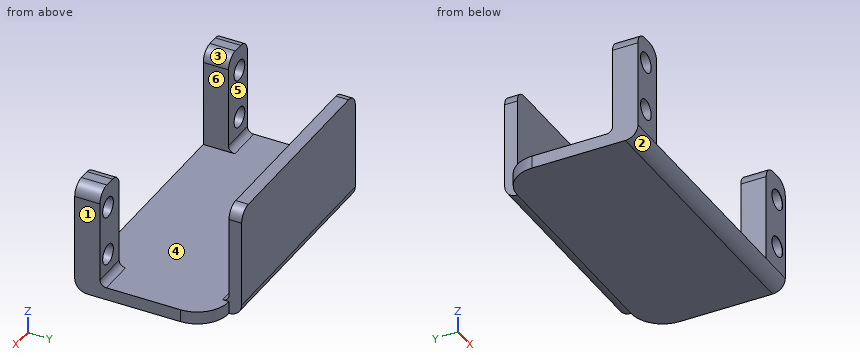
from build123d import *

# Parameters (mm, degrees)
SKETCH2_W                      = 42.8
SKETCH2_H                      = 2.54
BOSS_EXTRUDE1_DEPTH            = 2.54
SKETCH7_W                      = 7.192
SKETCH7_H                      = 5.08
SKETCH7_W_2                    = 42.8
SKETCH7_H_2                    = 2.54
BOSS_EXTRUDE3_DEPTH            = 20
FILLET3_R                      = 2.54
FILLET4_R                      = 1.27
CUT_EXTRUDE2_REACH             = 49.098
SKETCH8_R                      = 2.01
CUT_EXTRUDE2_DIRECTION_2_REACH = 49.098


# Some blends are built 0.0001 mm under size
with BuildPart() as part:
    # Sketch2 → Boss-Extrude1 (new body)
    with BuildSketch(Plane.XY):
        with Locations((-2.467346939, 15.826258503)):
            Rectangle(SKETCH2_W, SKETCH2_H)
        with BuildLine():
            Line((18.932653061, 14.556258503), (-23.867346939, 14.556258503))
            ThreePointArc((-23.867346939, 14.556258503), (-28.357474999, 12.696386564), (-30.217346939, 8.206258503))
            Line((-30.217346939, 8.206258503), (-30.217346939, -13.013741497))
            Line((-30.217346939, -13.013741497), (25.282653061, -13.013741497))
            Line((25.282653061, -13.013741497), (25.282653061, 8.206258503))
            ThreePointArc((25.282653061, 8.206258503), (23.422781122, 12.696386564), (18.932653061, 14.556258503))
        make_face()
    extrude(amount=-BOSS_EXTRUDE1_DEPTH)

    # Sketch7 → Boss-Extrude3 (add)
    with BuildSketch(Plane.XY):
        Polygon((-30.217346939, -7.933741497), (-30.217346939, -13.013741497), (-23.125346939, -13.003741497), (-23.125346939, -7.933741497), align=None)
        with Locations((21.686653061, -10.473741497)):
            Rectangle(SKETCH7_W, SKETCH7_H)
        with Locations((-2.467346939, 15.826258503)):
            Rectangle(SKETCH7_W_2, SKETCH7_H_2)
    extrude(amount=BOSS_EXTRUDE3_DEPTH)

    # Fillet3
    fillet3_edges = [part.edges().sort_by_distance(p)[0] for p in [
        (-2.467346939, 17.096258503, -2.54),
        (18.932653061, 15.826258503, 20),
        (-23.867346939, 15.826258503, 20),
        (-2.467346939, -13.013741497, -2.54),
        (18.090653061, -10.473741497, 20),
        (25.282653061, -10.473741497, 20),
        (-23.125346939, -10.468741497, 20),
        (-30.217346939, -10.473741497, 20),
    ]]
    fillet(fillet3_edges, radius=FILLET3_R - 0.0001)  # a hair under: the kernel refuses the full size

    # Fillet4
    # the kernel refuses this fillet: 1.27 mm, written as the material it adds along each edge
    with BuildSketch(Plane(origin=(-23.125346939, -7.933741497, 0), x_dir=(0, 1, 0), z_dir=(-1, 0, 0))) as fillet4_piece_1:
        with BuildLine():
            CenterArc((FILLET4_R, -FILLET4_R), FILLET4_R, 90, 90)
            Line((0, -FILLET4_R), (0, 0))
            Line((0, 0), (FILLET4_R, 0))
        make_face()
    extrude(amount=7.092)
    with BuildSketch(Plane(origin=(25.282653061, -7.933741497, 0), x_dir=(0, 1, 0), z_dir=(-1, 0, 0))) as fillet4_piece_2:
        with BuildLine():
            CenterArc((FILLET4_R, -FILLET4_R), FILLET4_R, 90, 90)
            Line((0, -FILLET4_R), (0, 0))
            Line((0, 0), (FILLET4_R, 0))
        make_face()
    extrude(amount=7.192)
    with BuildSketch(Plane(origin=(-23.867346939, 14.556258503, 0), x_dir=(0, 0, 1), z_dir=(1, 0, 0))) as fillet4_piece_3:
        with BuildLine():
            CenterArc((FILLET4_R, FILLET4_R), FILLET4_R, 180, 90)
            Line((0, FILLET4_R), (0, 0))
            Line((0, 0), (FILLET4_R, 0))
        make_face()
    extrude(amount=42.8)

    # Cut-Extrude2: up to this face of the body (flat: up to its plane)
    cut_extrude2_end = Plane(part.part.faces().sort_by_distance((-26.671346939, -7.933741497, 10.447713694))[0])
    # Sketch8 → Cut-Extrude2 (cut, up to the picked face)
    with BuildSketch(Plane(origin=(0.018289774, -12.971108055, 0), x_dir=(0.9999990058958133, 0.0014100380793790163, 0), z_dir=(0.0014100380793790163, -0.9999990058958133, 0)), mode=Mode.PRIVATE) as cut_extrude2_sk1:
        with Locations((-27.239885767, 5)):
            Circle(SKETCH8_R)
    cut_extrude2_tool1 = split(extrude(cut_extrude2_sk1.sketch, amount=-CUT_EXTRUDE2_REACH, mode=Mode.PRIVATE), bisect_by=cut_extrude2_end, keep=Keep.BOTH, mode=Mode.PRIVATE)
    # Sketch8 → Cut-Extrude2 (cut, up to the picked face)
    with BuildSketch(Plane(origin=(0.018289774, -12.971108055, 0), x_dir=(0.9999990058958133, 0.0014100380793790163, 0), z_dir=(0.0014100380793790163, -0.9999990058958133, 0)), mode=Mode.PRIVATE) as cut_extrude2_sk2:
        with Locations((22.260065025, 5)):
            Circle(SKETCH8_R)
    cut_extrude2_tool2 = split(extrude(cut_extrude2_sk2.sketch, amount=-CUT_EXTRUDE2_REACH, mode=Mode.PRIVATE), bisect_by=cut_extrude2_end, keep=Keep.BOTH, mode=Mode.PRIVATE)
    # Sketch8 → Cut-Extrude2 (cut, up to the picked face)
    with BuildSketch(Plane(origin=(0.018289774, -12.971108055, 0), x_dir=(0.9999990058958133, 0.0014100380793790163, 0), z_dir=(0.0014100380793790163, -0.9999990058958133, 0)), mode=Mode.PRIVATE) as cut_extrude2_sk3:
        with Locations((22.260065025, 15)):
            Circle(SKETCH8_R)
    cut_extrude2_tool3 = split(extrude(cut_extrude2_sk3.sketch, amount=-CUT_EXTRUDE2_REACH, mode=Mode.PRIVATE), bisect_by=cut_extrude2_end, keep=Keep.BOTH, mode=Mode.PRIVATE)
    # Sketch8 → Cut-Extrude2 (cut, up to the picked face)
    with BuildSketch(Plane(origin=(0.018289774, -12.971108055, 0), x_dir=(0.9999990058958133, 0.0014100380793790163, 0), z_dir=(0.0014100380793790163, -0.9999990058958133, 0)), mode=Mode.PRIVATE) as cut_extrude2_sk4:
        with Locations((-27.239885767, 15)):
            Circle(SKETCH8_R)
    cut_extrude2_tool4 = split(extrude(cut_extrude2_sk4.sketch, amount=-CUT_EXTRUDE2_REACH, mode=Mode.PRIVATE), bisect_by=cut_extrude2_end, keep=Keep.BOTH, mode=Mode.PRIVATE)
    add(cut_extrude2_tool1.solids().sort_by(Axis((-27.221569, -13.009517, 5), (-0.0014100380793790163, 0.9999990058958133, 0)))[0], mode=Mode.SUBTRACT)
    add(cut_extrude2_tool2.solids().sort_by(Axis((22.278333, -12.939721, 5), (-0.0014100380793790163, 0.9999990058958133, 0)))[0], mode=Mode.SUBTRACT)
    add(cut_extrude2_tool3.solids().sort_by(Axis((22.278333, -12.939721, 15), (-0.0014100380793790163, 0.9999990058958133, 0)))[0], mode=Mode.SUBTRACT)
    add(cut_extrude2_tool4.solids().sort_by(Axis((-27.221569, -13.009517, 15), (-0.0014100380793790163, 0.9999990058958133, 0)))[0], mode=Mode.SUBTRACT)

    # Cut-Extrude2 direction 2: up to this face of the body (flat: up to its plane)
    cut_extrude2_direction_2_end = Plane(part.part.faces().sort_by_distance((21.685702836, -13.013741497, 9.814476997))[0])
    # Sketch8 → Cut-Extrude2 direction 2 (cut, up to the picked face)
    with BuildSketch(Plane(origin=(0.018289774, -12.971108055, 0), x_dir=(0.9999990058958133, 0.0014100380793790163, 0), z_dir=(0.0014100380793790163, -0.9999990058958133, 0)), mode=Mode.PRIVATE) as cut_extrude2_direction_2_sk1:
        with Locations((-27.239885767, 5)):
            Circle(SKETCH8_R)
    cut_extrude2_direction_2_tool1 = split(extrude(cut_extrude2_direction_2_sk1.sketch, amount=CUT_EXTRUDE2_DIRECTION_2_REACH, mode=Mode.PRIVATE), bisect_by=cut_extrude2_direction_2_end, keep=Keep.BOTH, mode=Mode.PRIVATE)
    # Sketch8 → Cut-Extrude2 direction 2 (cut, up to the picked face)
    with BuildSketch(Plane(origin=(0.018289774, -12.971108055, 0), x_dir=(0.9999990058958133, 0.0014100380793790163, 0), z_dir=(0.0014100380793790163, -0.9999990058958133, 0)), mode=Mode.PRIVATE) as cut_extrude2_direction_2_sk2:
        with Locations((22.260065025, 5)):
            Circle(SKETCH8_R)
    cut_extrude2_direction_2_tool2 = split(extrude(cut_extrude2_direction_2_sk2.sketch, amount=CUT_EXTRUDE2_DIRECTION_2_REACH, mode=Mode.PRIVATE), bisect_by=cut_extrude2_direction_2_end, keep=Keep.BOTH, mode=Mode.PRIVATE)
    # Sketch8 → Cut-Extrude2 direction 2 (cut, up to the picked face)
    with BuildSketch(Plane(origin=(0.018289774, -12.971108055, 0), x_dir=(0.9999990058958133, 0.0014100380793790163, 0), z_dir=(0.0014100380793790163, -0.9999990058958133, 0)), mode=Mode.PRIVATE) as cut_extrude2_direction_2_sk3:
        with Locations((22.260065025, 15)):
            Circle(SKETCH8_R)
    cut_extrude2_direction_2_tool3 = split(extrude(cut_extrude2_direction_2_sk3.sketch, amount=CUT_EXTRUDE2_DIRECTION_2_REACH, mode=Mode.PRIVATE), bisect_by=cut_extrude2_direction_2_end, keep=Keep.BOTH, mode=Mode.PRIVATE)
    # Sketch8 → Cut-Extrude2 direction 2 (cut, up to the picked face)
    with BuildSketch(Plane(origin=(0.018289774, -12.971108055, 0), x_dir=(0.9999990058958133, 0.0014100380793790163, 0), z_dir=(0.0014100380793790163, -0.9999990058958133, 0)), mode=Mode.PRIVATE) as cut_extrude2_direction_2_sk4:
        with Locations((-27.239885767, 15)):
            Circle(SKETCH8_R)
    cut_extrude2_direction_2_tool4 = split(extrude(cut_extrude2_direction_2_sk4.sketch, amount=CUT_EXTRUDE2_DIRECTION_2_REACH, mode=Mode.PRIVATE), bisect_by=cut_extrude2_direction_2_end, keep=Keep.BOTH, mode=Mode.PRIVATE)
    add(cut_extrude2_direction_2_tool1.solids().sort_by(Axis((-27.221569, -13.009517, 5), (0.0014100380793790163, -0.9999990058958133, 0)))[0], mode=Mode.SUBTRACT)
    add(cut_extrude2_direction_2_tool2.solids().sort_by(Axis((22.278333, -12.939721, 5), (0.0014100380793790163, -0.9999990058958133, 0)))[0], mode=Mode.SUBTRACT)
    add(cut_extrude2_direction_2_tool3.solids().sort_by(Axis((22.278333, -12.939721, 15), (0.0014100380793790163, -0.9999990058958133, 0)))[0], mode=Mode.SUBTRACT)
    add(cut_extrude2_direction_2_tool4.solids().sort_by(Axis((-27.221569, -13.009517, 15), (0.0014100380793790163, -0.9999990058958133, 0)))[0], mode=Mode.SUBTRACT)


solid = part.part
Geometry check sheet. Reference: the model listing, model coordinates, mm. Face numbers are marked on the shaded views. A direction names the side the tool comes from. Round coordinates to 2 decimals unless told otherwise and drop trailing zeros. Write each loop counter-clockwise with the first axis right and the second up, starting at its lowest first coordinate (ties: lowest second). Pieces come first, ordered by that corner, then holes. Notation, with made-up numbers: (85.5, -22.5) - (97.5, -22.5) arc R20 ccw to (97.5, 14.5) - close; hole circle Ø4 at (43, 59.25). An arc over 180 degrees is marked (long way). One line per item, written item: value.
1. Cross-section at A-A on z = 9. Record the boundary of the cut face in (x, y).
The answers:
outline: (-30.22, -13.01) - (-23.13, -13) - (-23.13, -7.93) - (-30.22, -7.93) - close; (-23.87, 14.56) - (18.93, 14.56) - (18.93, 17.1) - (-23.87, 17.1) - close; (18.09, -13.01) - (25.28, -13.01) - (25.28, -7.93) - (18.09, -7.93) - close
2. Depth check by flat-ended pin: pin 1 Ø1 at (x, y) = (-21.5, -2) entering from +Z; pin 2 Ø1.1 at (y, z) = (16, 5) entering from +X; pin 3 Ø8 at (x, z) = (-28.5, 9.5) entering from +Y; pin 4 Ø1 at (y, z) = (13, 13.5) entering from +X. Enter the tip coordinate at first touch or a pass-through.
The answers:
pin 1: stops at z = 0
pin 2: stops at x = 18.93
pin 3: stops at y = -7.93
pin 4: passes through
3. Cross-section at C-C on z = 13.75. Record the boundary of the cut face in (x, y).
The answers:
outline: (-30.22, -13.01) - (-28.8, -13.01) - (-28.8, -7.93) - (-30.22, -7.93) - close; (-25.65, -13.01) - (-23.13, -13) - (-23.13, -7.93) - (-25.65, -7.93) - close; (-23.87, 14.56) - (18.93, 14.56) - (18.93, 17.1) - (-23.87, 17.1) - close; (18.09, -13.01) - (20.7, -13.01) - (20.7, -7.93) - (18.09, -7.93) - close; (23.85, -13.01) - (25.28, -13.01) - (25.28, -7.93) - (23.85, -7.93) - close
4. Scan lines: L1, parallel to X at y = -11, z = 10; L2, parallel to Z at x = 13, y = 11; L3, parallel to Y at x = -25, z = 1.5. Record each from-to range of solid material in increasing order.
The answers:
L1: x = -30.22 to -23.13, 18.09 to 25.28
L2: z = -2.54 to 0
L3: y = -13.01 to -7.93
5. Set-up check for the marked faces 4, 5 and 6: record each of +Z, -Z, +X, -X, +Y, -Y from which the full face is reachable in a straight line by a thin tool's end or side.
The answers:
face 4: +Z
face 5: +Z, +X, -X
face 6: +Z, -Y
6. Cross-section at D-D on y = -5. Record the boundary of the cut face in (x, z), and give its area (3 significant figures).
The answers:
outline: (-30.22, -2.54) - (25.28, -2.54) - (25.28, 0) - (-30.22, 0) - close
area: 141 mm^2
7. Mould release check, pull along X, two halves, no side actions. Record for the marked faces 1, 2 and 3: released by +X, released by -X, zero draft, split by the parting line, or undercut.
The answers:
face 1: released by +X
face 2: zero draft
face 3: undercut
